```python
from build123d import *

# Parameters (mm, degrees)
SKIZZE1_R                       = 2.7
AUFSATZ_LINEAR_AUSTRAGEN1_DEPTH = 2.95
SKIZZE2_R                       = 1.45
AUFSATZ_LINEAR_AUSTRAGEN2_DEPTH = 6
FASE1_SIZE                      = 0.3
SCHNITT_LINEAR_AUSTRAGEN1_DEPTH = 2.5


with BuildPart() as part:
    # Skizze1 → Aufsatz-Linear austragen1 (new body)
    with BuildSketch(Plane.XY):
        Circle(SKIZZE1_R)
    extrude(amount=AUFSATZ_LINEAR_AUSTRAGEN1_DEPTH)

    # Skizze2 → Aufsatz-Linear austragen2 (add)
    with BuildSketch(Plane.XY.offset(2.95)):
        Circle(SKIZZE2_R)
    extrude(amount=AUFSATZ_LINEAR_AUSTRAGEN2_DEPTH)

    # Fase1
    fase1_edges = [part.edges().sort_by_distance(p)[0] for p in [
        (-2.7, 0, 0),
        (-2.7, 0, 2.95),
        (-1.45, 0, 8.95),
    ]]
    chamfer(fase1_edges, length=FASE1_SIZE)

    # Skizze3 → Schnitt-Linear austragen1 (cut)
    with BuildSketch(Plane(origin=(0, 0, 0), x_dir=(-1, 0, 0), z_dir=(0, 0, -1))):
        Polygon((1.25, 0.721687836), (0, 1.443375673), (-1.25, 0.721687836), (-1.25, -0.721687836), (0, -1.443375673), (1.25, -0.721687836), align=None)
    extrude(amount=-SCHNITT_LINEAR_AUSTRAGEN1_DEPTH, mode=Mode.SUBTRACT)


solid = part.part
```
Model file for the job. Use its own axes, mm. A direction names the side the tool comes from. Coordinates: 2 decimals unless noted, no trailing zeros. Write each loop counter-clockwise with the first axis right and the second up, starting at its lowest first coordinate (ties: lowest second). Pieces come first, ordered by that corner, then holes. Notation, with made-up numbers: (-27, 36) - (-21, 36) arc R17 cw to (-21, 47) - close; hole circle Ø1 at (2.25, 57.25). An arc over 180 degrees is marked (long way). One line per question, with ' | ' between items. Start each with the question number.
Q1. Drill centre lines: line 1 (X direction, y = 0.1, z = 2.25); line 2 (Z direction, x = -0.1, y = 0); line 3 (Z direction, x = 0.6, y = 1.6). Where is each one in solid material? Low to high. Write a range as [from, to].
Q2. Cut at A-A, the plane y = 0. List the corners of the cut face in (x, z), then the cut area to 3 significant figures.
Q3. Cut at B-B, the plane z = 7.5. List the corners of the cut face in (x, y), then the cut area to 3 significant figures.
Q4. Pin check, flat tips, straight feed: pin 1 (3 mm diameter, centred on x = -1.5, y = 1.5, fed in from -Z); pin 2 (2 mm diameter, centred on x = -1, z = 3.5, fed in from +Y); pin 3 (3 mm diameter, centred on y = 1.5, z = 7.5, fed in from -X); pin 4 (1.2 mm diameter, centred on x = 0, y = -0.5, fed in from -Z). Stop position of each tip, or through.
Q5. 3-axis set-ups, long thin cutter, end or side, ignore diameter. For faces 4 (the face through (0, -2, 2.95)), 5 (the face through (1.03, -1.03, 0)), 6 (the face through (-0.616, -1.088, 1.232)): which of +Z, -Z, +X, -X, +Y, -Y reach the whole face in a straight line?
Q6. Pull direction X, two halves, no side cores. Call faces 1 (the face through (0, 0, 8.95)), 2 (the face through (-1.45, 0.06, 5.76)), 3 (the face through (0.616, 1.088, 1.232)): pulls with the +X half, pulls with the -X half, needs draft (parallel to the pull), parting line crosses it, or undercut.
Answer below:
1) line 1: [-2.7, -1.25], [1.25, 2.7] | line 2: [2.5, 8.95] | line 3: [0, 2.95]
2) outline: (-2.7, 0.3) - (-2.4, 0) - (-1.25, 0) - (-1.25, 2.5) - (1.25, 2.5) - (1.25, 0) - (2.4, 0) - (2.7, 0.3) - (2.7, 2.65) - (2.4, 2.95) - (1.45, 2.95) - (1.45, 8.65) - (1.15, 8.95) - (-1.15, 8.95) - (-1.45, 8.65) - (-1.45, 2.95) - (-2.4, 2.95) - (-2.7, 2.65) - close | area: 26.8 mm^2
3) outline: circle Ø2.9 at (0, 0) | area: 6.61 mm^2
4) pin 1: z = 0 | pin 2: y = 2.66 | pin 3: x = -1.45 | pin 4: z = 2.5
5) face 4: +Z | face 5: -Z, +X, -X, +Y, -Y | face 6: -Z
6) face 1: needs draft | face 2: parting line crosses it | face 3: undercut
